Source: CAD feature listing. Evaluate the final solid. Frame: model axes, mm. Face numbers are marked on the shaded views. A direction names the side the tool comes from. Round coordinates to 2 decimals unless told otherwise and drop trailing zeros. Order: outer loops, then holes, each group sorted by start corner. A loop starts at its lowest first (then second) coordinate and runs counter-clockwise, first axis right, second up.
```python
from build123d import *

# Parameters (mm, degrees)
HEAD_DEPTH = 3
SKETCH3_R  = 0.25
PINS_DEPTH = 15


with BuildPart() as part:
    # Sketch2 → Head (new body)
    with BuildSketch(Plane(origin=(0, 0, 0), x_dir=(1, 0, 0), z_dir=(0, 1, 0))):
        Polygon((-2, 0), (-2, 1), (2, 1), (2, 0), (2, -1), (-2, -1), align=None)
    extrude(amount=HEAD_DEPTH)

    # Sketch3 → Pins (add)
    with BuildSketch(Plane(origin=(0, 0, 0), x_dir=(1, 0, 0), z_dir=(0, 1, 0))):
        with Locations(Location((0, 0, 0), (0, 0, 270))):
            Circle(SKETCH3_R)
        with Locations(Location((-1, 0, 0), (0, 0, 270))):
            Circle(SKETCH3_R)
        with Locations(Location((1, 0, 0), (0, 0, 270))):
            Circle(SKETCH3_R)
    extrude(amount=-PINS_DEPTH)


solid = part.part
```
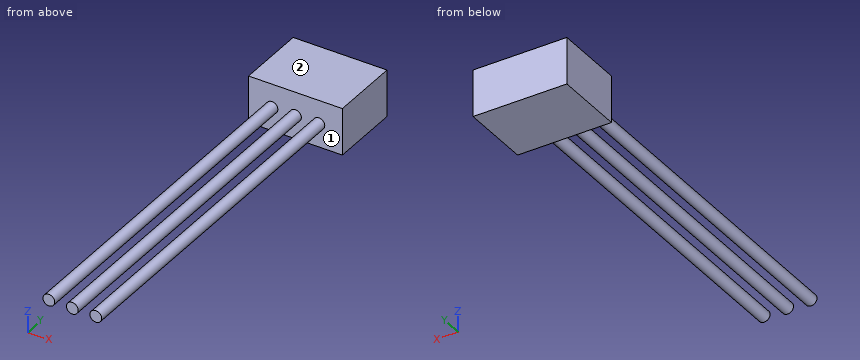
1. Section B-B on x = 0. Return loops of the section in (y, z), plus the area to 3 significant figures.
2. Access query for the marked faces 1 and 2. Directions: +Z, -Z, +X, -X, +Y, -Y. A direction counts if a zero-diameter tool reaches every point of the face in a straight line with its end or side. Return the directions, or none.
3. Section D-D on x = -1.5. Return loops of the section in (y, z), plus the area to 3 significant figures.
4. Section C-C on y = -8. Return loops of the section in (x, z), plus the area to 3 significant figures.
5. Line query: line 1 along X through (y, z) = (-8.5, -0.2); line 2 along Y through (x, z) = (1.8, -0.15); line 3 along Z through (x, y) = (1.05, -10.75). Output: solid intervals per line, ascending.
6. Section A-A on z = 0. Return loops of the section in (x, y), plus the area to 3 significant figures.
7. First-contact query: pin 1 (1.5 mm diameter, centred on x = 0, y = -0.5, fed in from -Z). Flat tip, straight axial feed; report the tip coordinate or a pass-through.
Result:
1. outline: (-15, -0.25) - (0, -0.25) - (0, -1) - (3, -1) - (3, 1) - (0, 1) - (0, 0.25) - (-15, 0.25) - close
1. area: 13.5 mm2
2. face 1: -Y
2. face 2: +Z, +X, -X, +Y, -Y
3. outline: (0, -1) - (3, -1) - (3, 1) - (0, 1) - close
3. area: 6.00 mm2
4. outline: circle Ø0.5 at (-1, 0); circle Ø0.5 at (0, 0); circle Ø0.5 at (1, 0)
4. area: 0.589 mm2
5. line 1: x = -1.15 to -0.85, -0.15 to 0.15, 0.85 to 1.15
5. line 2: y = 0 to 3
5. line 3: z = -0.24 to 0.24
6. outline: (-2, 0) - (-1.25, 0) - (-1.25, -15) - (-0.75, -15) - (-0.75, 0) - (-0.25, 0) - (-0.25, -15) - (0.25, -15) - (0.25, 0) - (0.75, 0) - (0.75, -15) - (1.25, -15) - (1.25, 0) - (2, 0) - (2, 3) - (-2, 3) - close
6. area: 34.5 mm2
7. pin 1: stops at z = -1
